Read the model definition and answer for the solid it produces. Units are mm, in the model's axes. A direction names the side the tool comes from. Round coordinates to 2 decimals unless told otherwise and drop trailing zeros. Loops run counter-clockwise (first coordinate to the right, second up) from the corner with the lowest first, then second, coordinate; pieces in that order, holes last. Notation, with made-up numbers: (-11, 33) - (-6, 33) arc R17 cw to (-6, 57) - close; hole circle Ø1 at (-35, -2.5). An arc over 180 degrees is marked (long way). Use one line per item in the form item = value. Start each with the question number.
```python
from build123d import *

# Parameters (mm, degrees)
F1_W     = 120
F1_H     = 40
F2_DEPTH = 40
F1_W_2   = 4
F3_DEPTH = 80
F4_R     = 5


with BuildPart() as f2:
    # F1 (on Top) → F2 (new body)
    with BuildSketch(Plane.XY):
        with Locations((-60, -20)):
            Rectangle(F1_W, F1_H)
    extrude(amount=F2_DEPTH)

    # F1 (on Top) → F3 (join)
    with BuildSketch(Plane.XY):
        with Locations((2, -20)):
            Rectangle(F1_W_2, F1_H)
        with Locations((-122, -20)):
            Rectangle(F1_W_2, F1_H)
    extrude(amount=F3_DEPTH)

    # F4
    f4_edges = [f2.edges().sort_by_distance(p)[0] for p in [
        (-60, -40, 40),
        (-60, 0, 40),
        (-122, -40, 80),
        (-122, 0, 80),
        (2, -40, 80),
        (2, 0, 80),
    ]]
    fillet(f4_edges, radius=F4_R)


solid = f2.part
```
1) Flat-ended cylindrical pins translate along their axes: pin 1 (3 mm diameter, centred on x = -42.5, y = -23, fed in from +Z); pin 2 (6 mm diameter, centred on x = -38, y = -30.5, fed in from -Z). Find the tip coordinate at first contact, or state that the pin passes through.
2) Determine the mould class of faces 1 (the flat face through (-61, -20, 40)), 2 (the flat face through (-61, -20, 0)), 3 (the flat face through (4, -20, 39)) for opening direction X: +X half, -X half, draft (parallel to the pull), parting line (faces both ways), or undercut.
3) A cutting plane is placed at B-B on y = -30. Write down the section's boundary in (x, z).
4) A cutting plane is placed at C-C on x = -82.5. Write down the section's boundary in (y, z), plus the area to 3 significant figures.
5) For faces 4 (the cylindrical face through (-59, -1, 38)), 5 (the cylindrical face through (-59, -39, 38)), 6 (the flat face through (-61, -40, 12)), determine the directions among +Z, -Z, +X, -X, +Y, -Y from which every point of the face is accessible in a straight line to the end or side of a thin tool.
6) Straight lines are drawn through the part: line 1 (X direction, y = -38, z = 46.5); line 2 (Z direction, x = -21.5, y = -35.5); line 3 (Z direction, x = -99, y = -4). For each, find the intervals that lie inside material, in ascending order. Write a range as from..to.
7) A cutting plane is placed at A-A on z = 61.5. Write down the section's boundary in (x, y), plus the area to 3 significant figures.
Checks:
q1.pin_1 = 40
q1.pin_2 = 0
q2.face_1 = undercut
q2.face_2 = draft
q2.face_3 = +X half
q3.outline = (-124, 0) - (4, 0) - (4, 80) - (0, 80) - (0, 40) - (-120, 40) - (-120, 80) - (-124, 80) - close
q4.outline = (-40, 0) - (0, 0) - (0, 35) arc R5 ccw to (-5, 40) - (-35, 40) arc R5 ccw to (-40, 35) - close
q4.area = 1,590 mm²
q5.face_4 = +Z, +Y
q5.face_5 = +Z, -Y
q5.face_6 = +Z, -Z, +X, -X, -Y
q6.line_1 = -124..-120, 0..4
q6.line_2 = 0..39.97
q6.line_3 = 0..39.9
q7.outline = (-124, -40) - (-120, -40) - (-120, 0) - (-124, 0) - close; (0, -40) - (4, -40) - (4, 0) - (0, 0) - close
q7.area = 320 mm²
